```python
from build123d import *

# Parameters (mm, degrees)
SKETCH006_R            = 14.2875
PAD006_DEPTH           = 273.05
SKETCH007_W            = 57.15
SKETCH007_H            = 57.15
PAD007_DEPTH           = 28.575
SKETCH008_R            = 12.7
PAD008_DEPTH           = 9.525
LINEARPATTERN001_COUNT = 2
LINEARPATTERN001_PITCH = 47.625
SKETCH010_R            = 7.9375
PAD010_DEPTH           = 257.175
ARRAY_X_COUNT          = 2
ARRAY_X_PITCH          = 54.61
ARRAY_Y_COUNT          = 2
ARRAY_Y_PITCH          = 54.61
SKETCH_W               = 76.2
SKETCH_H               = 76.2
SKETCH_R               = 7.9375
PAD_DEPTH              = 12.7
PAD001_DEPTH           = 14.2875
SKETCH002_R            = 12.7
PAD002_DEPTH           = 15.875
LINEARPATTERN_COUNT    = 2
LINEARPATTERN_PITCH    = 44.45
SKETCH003_R            = 28.575
SKETCH003_R_2          = 25.4
PAD003_DEPTH           = 203.2
SKETCH004_W            = 76.2
SKETCH004_H            = 76.2
SKETCH004_R            = 7.9375
SKETCH004_R_2          = 25.4
PAD004_DEPTH           = 12.7
SKETCH005_R            = 14.2875
PAD005_DEPTH           = 17.145
CYLINDER_R             = 12.7
CYLINDER_DEPTH         = 101.6
CYLINDER_ROLL_ANGLE    = 90


with BuildPart() as body001:
    # Sketch006 → Pad006 (new body)
    with BuildSketch(Plane.XY):
        Circle(SKETCH006_R)
    extrude(amount=-PAD006_DEPTH)

    # Sketch007 (on Face3 of Pad006) → Pad007 (join)
    with BuildSketch(Plane(origin=(0, 0, -273.05), x_dir=(1, 0, 0), z_dir=(0, 0, -1))):
        Rectangle(SKETCH007_W, SKETCH007_H)
    extrude(amount=-PAD007_DEPTH)

    # Sketch008 (on Face4 of Pad007) → Pad008 (join)
    with BuildSketch(Plane.XZ.offset(28.575)):
        with BuildLine():
            Line((-25.4, -247.65), (25.4, -247.65))
            Line((25.4, -247.65), (25.4, -328.929945))
            ThreePointArc((-25.4, -328.929945), (0, -354.33), (25.4, -328.929945))
            Line((-25.4, -328.929945), (-25.4, -247.65))
        make_face()
        with Locations((0, -328.93)):
            Circle(SKETCH008_R, mode=Mode.SUBTRACT)
    pad008 = extrude(amount=-PAD008_DEPTH)

    # LinearPattern001: Pad008 ×2
    with Locations(*[(0, i * LINEARPATTERN001_PITCH, 0) for i in range(1, LINEARPATTERN001_COUNT)]):
        add(pad008)


with BuildPart() as array:
    # Sketch010 → Pad010 (new body)
    with BuildSketch(Plane.XY):
        with Locations((26.9875, -26.9875)):
            Circle(SKETCH010_R)
    extrude(amount=-PAD010_DEPTH)

    # Array X: Array ×2


with BuildPart() as array_1:
    add(array.part)
    with Locations(*[(-i * ARRAY_X_PITCH, 0, 0) for i in range(1, ARRAY_X_COUNT)]):
        add(array.part)

    # Array Y: Array ×2


with BuildPart() as array_2:
    add(array_1.part)
    with Locations(*[(0, i * ARRAY_Y_PITCH, 0) for i in range(1, ARRAY_Y_COUNT)]):
        add(array_1.part)


with BuildPart() as array_3:
    # Array placement: moved
    add(array_2.part.moved(Location((0, 0, 25.4))))


with BuildPart() as fusion:
    # Sketch → Pad (new body)
    with BuildSketch(Plane.XY):
        Rectangle(SKETCH_W, SKETCH_H)
        with Locations((-26.9875, 26.9875)):
            Circle(SKETCH_R, mode=Mode.SUBTRACT)
        with Locations((26.9875, 26.9875)):
            Circle(SKETCH_R, mode=Mode.SUBTRACT)
        with Locations((-26.9875, -26.9875)):
            Circle(SKETCH_R, mode=Mode.SUBTRACT)
        with Locations((26.9875, -26.9875)):
            Circle(SKETCH_R, mode=Mode.SUBTRACT)
    extrude(amount=PAD_DEPTH)

    # Sketch001 → Pad001 (join, symmetric)
    with BuildSketch(Plane(origin=(0, 0, 12.7), x_dir=(1, 0, 0), z_dir=(0, -1, 0))):
        Polygon((-38.1, 0), (38.1, 0), (22.225, 19.05), (-22.225, 19.05), align=None)
    extrude(amount=PAD001_DEPTH, both=True)

    # Sketch002 (on Face15 of Pad001) → Pad002 (join)
    with BuildSketch(Plane.XZ.offset(14.2875)):
        with BuildLine():
            Line((-17.4625, 0), (17.4625, 0))
            Line((17.4625, 0), (17.4625, 65.374917))
            ThreePointArc((17.4625, 65.374917), (0, 109.22), (-17.4625, 65.374917))
            Line((-17.4625, 65.374917), (-17.4625, 0))
        make_face()
        with Locations((0, 83.82)):
            Circle(SKETCH002_R, mode=Mode.SUBTRACT)
    pad002 = extrude(amount=PAD002_DEPTH)

    # LinearPattern: Pad002 ×2
    with Locations(*[(0, i * LINEARPATTERN_PITCH, 0) for i in range(1, LINEARPATTERN_COUNT)]):
        add(pad002)

    # Sketch003 (on Face4 of LinearPattern) → Pad003 (join)
    with BuildSketch(Plane(origin=(0, 0, 0), x_dir=(1, 0, 0), z_dir=(0, 0, -1))):
        Circle(SKETCH003_R)
        Circle(SKETCH003_R_2, mode=Mode.SUBTRACT)
    extrude(amount=PAD003_DEPTH)

    # Sketch004 (on Face28 of Pad003) → Pad004 (join)
    with BuildSketch(Plane(origin=(0, 0, -203.2), x_dir=(1, 0, 0), z_dir=(0, 0, -1))):
        Rectangle(SKETCH004_W, SKETCH004_H)
        with Locations((-26.9875, 26.9875)):
            Circle(SKETCH004_R, mode=Mode.SUBTRACT)
        with Locations((26.9875, 26.9875)):
            Circle(SKETCH004_R, mode=Mode.SUBTRACT)
        with Locations((-26.9875, -26.9875)):
            Circle(SKETCH004_R, mode=Mode.SUBTRACT)
        with Locations((26.9875, -26.9875)):
            Circle(SKETCH004_R, mode=Mode.SUBTRACT)
        Circle(SKETCH004_R_2, mode=Mode.SUBTRACT)
    extrude(amount=PAD004_DEPTH)

    # Sketch005 (on Face43 of Pad004) → Pad005 (join)
    with BuildSketch(Plane(origin=(0, 0, -215.9), x_dir=(1, 0, 0), z_dir=(0, 0, -1))):
        with BuildLine():
            ThreePointArc((21.997045, 12.7), (17.960512, 17.960512), (12.7, 21.997045))
            Line((12.7, 34.697045), (12.7, 21.997045))
            Line((-12.7, 34.697045), (12.7, 34.697045))
            Line((-12.7, 21.997045), (-12.7, 34.697045))
            ThreePointArc((-12.7, 21.997045), (-17.960512, 17.960512), (-21.997045, 12.7))
            Line((-34.697045, 12.7), (-21.997045, 12.7))
            Line((-34.697045, -12.7), (-34.697045, 12.7))
            Line((-21.997045, -12.7), (-34.697045, -12.7))
            ThreePointArc((-21.997045, -12.7), (-17.960512, -17.960512), (-12.7, -21.997045))
            Line((-12.7, -21.997045), (-12.7, -47.397045))
            Line((-12.7, -47.397045), (12.7, -47.397045))
            Line((12.7, -47.397045), (12.7, -21.997045))
            ThreePointArc((12.7, -21.997045), (17.960512, -17.960512), (21.997045, -12.7))
            Line((21.997045, -12.7), (34.697045, -12.7))
            Line((34.697045, -12.7), (34.697045, 12.7))
            Line((34.697045, 12.7), (21.997045, 12.7))
        make_face()
        Circle(SKETCH005_R, mode=Mode.SUBTRACT)
    extrude(amount=PAD005_DEPTH)

    # Fusion: union Body001, Array
    add(body001.part)
    add(array_3.part)


with BuildPart() as cylinder:
    # Cylinder → Cylinder (new body)
    with BuildSketch(Plane.XY):
        Circle(CYLINDER_R)
    extrude(amount=CYLINDER_DEPTH)


with BuildPart() as cylinder_1:
    # Cylinder roll: moved
    add(cylinder.part.rotate(Axis((0, 0, 0), (1, 0, 0)), CYLINDER_ROLL_ANGLE))


with BuildPart() as cylinder_2:
    # Cylinder placement: moved
    add(cylinder_1.part.moved(Location((0, 50.8, 83.82))))


with BuildPart() as cylinder001:
    # Clone base: copy of Cylinder
    add(cylinder_2.part)


with BuildPart() as cylinder001_1:
    # Clone placement: moved
    add(cylinder001.part.moved(Location((0, 0, -412.75))))


with BuildPart() as fusion001:
    # Fusion001 base: copy of Cylinder
    add(cylinder_2.part)

    # Fusion001: union Fusion, Cylinder001
    add(fusion.part)
    add(cylinder001_1.part)


solid = fusion001.part
```
Work out the finished part from the listing and answer in its coordinate system (mm). A direction names the side the tool comes from. Round coordinates to 2 decimals unless told otherwise and drop trailing zeros. Write each loop counter-clockwise with the first axis right and the second up, starting at its lowest first coordinate (ties: lowest second). Pieces come first, ordered by that corner, then holes. Notation, with made-up numbers: (5.25, 56.5) - (61.25, 56.5) arc R23 ccw to (61.25, 89.5) - close; hole circle Ø6 at (50, 30). An arc over 180 degrees is marked (long way). Return JSON: item names as keys, results as strings. Group by question number.
Q1. The part is cut by section A-A on z = -195. Count the separate pieces of the cut face and the enclosed holes in it, then the cut area to 3 significant figures.
Q2. Each of these flat-tipped pins is pushed along its axis until it touches: pin 1 Ø8 at (x, y) = (5.5, -11) entering from +Z; pin 2 Ø21 at (x, y) = (-7, -12.5) entering from -Z; pin 3 Ø8 at (x, y) = (-8, 28.5) entering from +Z. Where does it stop, or does it pass through?
Q3. Find the intervals of material crossed by L1, parallel to X at y = 0, z = -165 (1 decimal); L2, parallel to Z at x = 14.5, y = -2.5 (3 decimals); L3, parallel to Z at x = -0.5, y = -6.5, in increasing order.
Q4. The part is cut by section C-C on z = 83.82. Write down the section's boundary in (x, y), then the cut area to 3 significant figures.
Q5. The mould has two halves that part along Z. Classify faces 1 (the flat face through (-25.4, 24, -301)), 2 (the cylindrical face through (-0.559, -23.879, -354.324)), 3 (the flat face through (25, -14.288, 20)): released by +Z, released by -Z, zero draft, split by the parting line, or undercut.
Q6. For faces 4 (the flat face through (16, -26, -203.2)), 5 (the cylindrical face through (6.827, 40.626, 94.529)), 6 (the flat face through (-26, -14.288, 20)), determine the directions among +Z, -Z, +X, -X, +Y, -Y from which every point of the face is accessible in a straight line to the end or side of a thin tool.
Solved:
{
 "1": {"separate pieces": "6", "enclosed holes": "1", "area": "1,970 mm²"},
 "2": {"pin 1": "z = 109.01", "pin 2": "z = -354.33", "pin 3": "z = 108.9"},
 "3": {"L1": "-28.6 to -25.4, -14.3 to 14.3, 25.4 to 28.6", "L2": "-273.05 to -244.475, -233.045 to -215.9, 0 to 31.75", "L3": "-341.62 to -316.24, -273.05 to 31.75, 71.13 to 96.51"},
 "4": {"outline": "(-25.4, -30.16) - (-12.7, -30.16) - (-12.7, -50.8) - (12.7, -50.8) - (12.7, -30.16) - (25.4, -30.16) - (25.4, -14.29) - (12.7, -14.29) - (12.7, 14.29) - (25.4, 14.29) - (25.4, 30.16) - (12.7, 30.16) - (12.7, 50.8) - (-12.7, 50.8) - (-12.7, 30.16) - (-25.4, 30.16) - (-25.4, 14.29) - (-12.7, 14.29) - (-12.7, -14.29) - (-25.4, -14.29) - close", "area": "3,390 mm²"},
 "5": {"face 1": "zero draft", "face 2": "released by -Z", "face 3": "undercut"},
 "6": {"face 4": "none", "face 5": "+Y", "face 6": "-X"}
}
